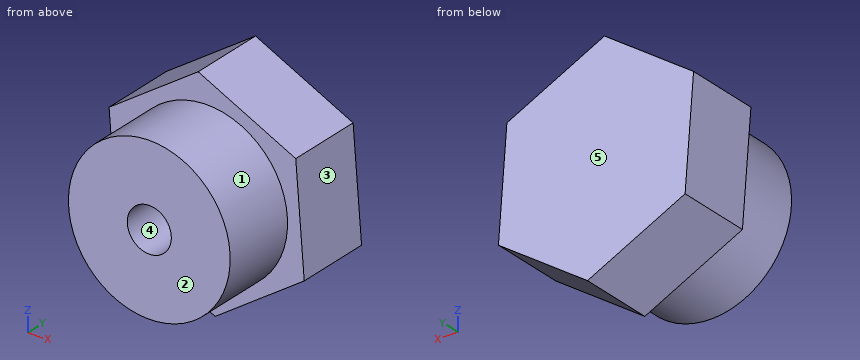
Autodesk Inventor part; units mm, degrees
ref_plane "YZ Plane" through (0, 0, 0) normal (1, 0, 0) x (0, 1, 0)
ref_plane "XZ Plane" through (0, 0, 0) normal (0, 1, 0) x (-1, 0, 0)
ref_plane "XY Plane" through (0, 0, 0) normal (0, 0, 1) x (1, 0, 0)
sketch "Sketch1" plane through (0, 0, 0) normal (0, 1, 0) x (-1, 0, 0)
  circle A0 centre (0, 0) radius 10.7576
extrude "Extrusion1" add sketch "Sketch1" along normal blind 10
sketch "Sketch2" plane through (0, 10, 0) normal (0, 1, 0) x (1, 0, 0)
  circle A0 centre (0, 0) radius 10.7576
  circle A1 centre (0, 0) radius 2.9303
extrude "Extrusion2" cut sketch "Sketch2" against normal blind 10 contours A1
sketch "Sketch3" plane through (0, 10, 0) normal (0, 1, 0) x (1, 0, 0)
  line L0 (11.8466, -8.1445) -> (-1.1301, -14.3317)
  line L1 (-1.1301, -14.3317) -> (-12.9767, -6.1872)
  line L2 (-12.9767, -6.1872) -> (-11.8466, 8.1445)
  line L3 (-11.8466, 8.1445) -> (1.1301, 14.3317)
  line L4 (1.1301, 14.3317) -> (12.9767, 6.1872)
  line L5 (12.9767, 6.1872) -> (11.8466, -8.1445)
  point P0 (0, 0)
  point P1 (0, 0)
extrude "Extrusion3" add sketch "Sketch3" along normal blind 10
The listing builds one solid part. Answer for the finished solid, in the listing's coordinates (mm). Face numbers are marked on the shaded views. A direction names the side the tool comes from. Round coordinates to 2 decimals unless told otherwise and drop trailing zeros. Loops run counter-clockwise (first coordinate to the right, second up) from the corner with the lowest first, then second, coordinate; pieces in that order, holes last.
1) For a pull along X with two mould halves and no side action, classify the marked faces 3, 4 and 5 as released by +X, released by -X, zero draft, split by the parting line, or undercut.
Outcome:
face 3: released by +X
face 4: undercut
face 5: zero draft
2) A cutting plane is placed at C-C on x = 2.5. Determine the outline of the cut face in (y, z).
Outcome:
outline: (0, -10.46) - (10, -10.46) - (10, -13.39) - (20, -13.39) - (20, 12.6) - (10, 12.6) - (10, 10.46) - (0, 10.46) - (0, 1.53) - (10, 1.53) - (10, -1.53) - (0, -1.53) - close
3) Given P1, Ø3, axis at x = 3, y = 13, coming from the +Z side; P2, Ø8, axis at y = 11.5, z = 4.5, coming from the +X side; P3, Ø8, axis at y = 13.5, z = -2, coming from the -X side, each flat-ended and moving along its own axis, determine where each tip first touches the part or whether it passes through.
Outcome:
P1: stops at z = 13.08
P2: stops at x = 12.45
P3: stops at x = -12.65
4) A cutting plane is placed at A-A on y = 10.5. Determine the outline of the cut face in (x, z), plus the area to 3 significant figures.
Outcome:
outline: (-12.98, 6.19) - (-11.85, -8.14) - (1.13, -14.33) - (12.98, -6.19) - (11.85, 8.14) - (-1.13, 14.33) - close
area: 537 mm2
5) Consider line 1 (Z direction, x = 0, y = 5.75); line 2 (Y direction, x = -11.5, z = 0.5); line 3 (Z direction, x = -5.25, y = 6.75). Determine where each line is inside the solid, lowest interval first.
Outcome:
line 1: z = -10.76 to -2.93, 2.93 to 10.76
line 2: y = 10 to 20
line 3: z = -9.39 to 9.39
6) For the marked faces 1 and 2, determine the directions among +Z, -Z, +X, -X, +Y, -Y from which every point of the face is accessible in a straight line to the end or side of a thin tool.
Outcome:
face 1: -Y
face 2: +Z, -Z, +X, -X, -Y
7) A cutting plane is placed at D-D on y = 7.75. Determine the outline of the cut face in (x, z).
Outcome:
outline: circle Ø21.52 at (0, 0); hole circle Ø5.86 at (0, 0)
8) A cutting plane is placed at B-B on z = 7.5. Determine the outline of the cut face in (x, y).
Outcome:
outline: (-11.07, 10) - (-7.71, 10) - (-7.71, 0) - (7.71, 0) - (7.71, 10) - (11.9, 10) - (11.9, 20) - (-11.07, 20) - close
